Source: CAD feature listing. Evaluate the final solid. Frame: model axes, mm. A direction names the side the tool comes from. Round coordinates to 2 decimals unless told otherwise and drop trailing zeros. Write each loop counter-clockwise with the first axis right and the second up, starting at its lowest first coordinate (ties: lowest second). Pieces come first, ordered by that corner, then holes.
```python
from build123d import *

# Parameters (mm, degrees)
SKETCH1_R           = 2.7
BOSS_EXTRUDE1_DEPTH = 4
CHAMFER1_SIZE       = 1
SKETCH3_R           = 2.4
CUT_EXTRUDE1_DEPTH  = 7
CHAMFER2_SIZE       = 0.5


with BuildPart() as part:
    # Sketch1 → Boss-Extrude1 (new, symmetric)
    with BuildSketch(Plane(origin=(0, 0, 0), x_dir=(0, 0, -1), z_dir=(1, 0, 0))):
        with BuildLine():
            Line((-4.451593815, 2.276688935), (-10.670956289, -9.883986639))
            ThreePointArc((-10.670956289, -9.883986639), (-10.559105321, -12.815560589), (-8, -14.25))
            Line((-8, -14.25), (8, -14.25))
            ThreePointArc((8, -14.25), (10.559105321, -12.815560589), (10.670956289, -9.883986639))
            Line((10.670956289, -9.883986639), (4.451593815, 2.276688935))
            ThreePointArc((4.451593815, 2.276688935), (0, 5), (-4.451593815, 2.276688935))
        make_face()
        Circle(SKETCH1_R, mode=Mode.SUBTRACT)
    extrude(amount=BOSS_EXTRUDE1_DEPTH, both=True)

    # Chamfer1
    chamfer1_edges = [part.edges().sort_by_distance(p)[0] for p in [
        (4, -12.815560589, 10.559105321),
        (4, -14.25, 0),
        (4, -12.815560589, -10.559105321),
        (4, -3.803648852, -7.561275052),
        (4, 5, 0),
        (-4, -3.803648852, -7.561275052),
        (-4, -12.815560589, -10.559105321),
        (-4, -14.25, 0),
        (-4, -12.815560589, 10.559105321),
        (-4, -3.803648852, 7.561275052),
        (-4, 5, 0),
        (4, -3.803648852, 7.561275052),
    ]]
    chamfer(chamfer1_edges, length=CHAMFER1_SIZE)

    # Sketch3 → Cut-Extrude1 (cut)
    with BuildSketch(Plane.XZ.offset(14.25)):
        with Locations(Location((0, 5, 0), (0, 0, 270))):
            Circle(SKETCH3_R)
        with Locations(Location((0, -5, 0), (0, 0, 270))):
            Circle(SKETCH3_R)
    extrude(amount=-CUT_EXTRUDE1_DEPTH, mode=Mode.SUBTRACT)

    # Chamfer2
    chamfer2_edges = [part.edges().sort_by_distance(p)[0] for p in [
        (0, -14.25, 7.4),
        (0, -14.25, -2.6),
    ]]
    chamfer(chamfer2_edges, length=CHAMFER2_SIZE)


solid = part.part
```
Q1. Section query B-B, the plane x = 0. Output: boundary loops of the cut face in (y, z), and give its area (3 significant figures).
Q2. Section query D-D, the plane y = -3.25. Output: boundary loops of the cut face in (x, z), and give its area (3 significant figures).
Q3. Mould query, pull axis Y, two halves, no side actions, for faces 1 (the face through (0.04, -12.78, 10.58)), 2 (the face through (-0.056, -2.636, 0.585)), 3 (the face through (0, -14.25, 0)), 4 (the face through (3.49, -3.94, 7.08)). Classes: pulls with the +Y half, pulls with the -Y half, needs draft (parallel to the pull), parting line crosses it, or undercut.
Q4. Line query: line 1 (X direction, y = -10, z = 5); line 2 (Y direction, x = 1.5, z = 0); line 3 (Z direction, x = 0, y = -1.25). Output: solid intervals per line, ascending.
Q5. Section query A-A, the plane z = 0. Output: boundary loops of the cut face in (x, y), and give its area (3 significant figures).
Q6. Pin query (flat end, axial travel): P1, Ø4.5, axis at x = 0, z = -5, coming from the -Y side; P2, Ø2, axis at x = -1.5, z = -4.5, coming from the -Y side. Return the tip coordinate at first contact, or that it passes through.
Q7. Set-up query: faces 5 (the face through (-3.507, -3.949, 7.066)), 6 (the face through (0, -7.25, -5)). Return all of +Z, -Z, +X, -X, +Y, -Y with unobstructed straight access to the full face (end or side cutting, diameter ignored); none if empty.
Q8. Section query C-C, the plane y = 0. Output: boundary loops of the cut face in (x, z).
Filled in:
1. outline: (-14.25, -8) arc R3 ccw to (-9.88, -10.67) - (2.28, -4.45) arc R5 ccw to (2.28, 4.45) - (-9.88, 10.67) arc R3 ccw to (-14.25, 8) - (-14.25, 7.9) - (-13.75, 7.4) - (-7.25, 7.4) - (-7.25, 2.6) - (-13.75, 2.6) - (-14.25, 2.1) - (-14.25, -2.1) - (-13.75, -2.6) - (-7.25, -2.6) - (-7.25, -7.4) - (-13.75, -7.4) - (-14.25, -7.9) - close; hole circle Ø5.4 at (0, 0)
1. area: 203 mm2
2. outline: (-4, -6.15) - (-3, -7.28) - (3, -7.28) - (4, -6.15) - (4, 6.15) - (3, 7.28) - (-3, 7.28) - (-4, 6.15) - close
2. area: 114 mm2
3. face 1: parting line crosses it
3. face 2: undercut
3. face 3: pulls with the -Y half
3. face 4: pulls with the +Y half
4. line 1: x = -4 to -2.4, 2.4 to 4
4. line 2: y = -14.25 to -2.7, 2.7 to 5
4. line 3: z = -6.26 to -2.39, 2.39 to 6.26
5. outline: (-4, -13.25) - (-3, -14.25) - (3, -14.25) - (4, -13.25) - (4, -2.7) - (-4, -2.7) - close; (-4, 2.7) - (4, 2.7) - (4, 4) - (3, 5) - (-3, 5) - (-4, 4) - close
5. area: 109 mm2
6. P1: stops at y = -7.25
6. P2: stops at y = -13.93
7. face 5: +Z, -X, +Y
7. face 6: -Y
8. outline: (-4, -4.49) - (-3, -5.62) - (3, -5.62) - (4, -4.49) - (4, -2.7) - (-4, -2.7) - close; (-4, 2.7) - (4, 2.7) - (4, 4.49) - (3, 5.62) - (-3, 5.62) - (-4, 4.49) - close
